```python
from build123d import *

# Parameters (mm, degrees)
SKETCH1_W           = 127
SKETCH1_H           = 127
BOSS_EXTRUDE1_DEPTH = 6.35
SKETCH2_W           = 50.8
SKETCH2_H           = 63.5
CUT_EXTRUDE1_DEPTH  = 180.717340566
SKETCH3_R           = 14.3002
CUT_EXTRUDE2_DEPTH  = 180.717340566
SKETCH5_R           = 2.5527
CUT_EXTRUDE4_DEPTH  = 180.717340566
CIRPATTERN1_COUNT   = 8
SKETCH6_R           = 14.3002
CUT_EXTRUDE5_DEPTH  = 180.717340566
FILLET1_R           = 2.54
FILLET2_R           = 25.4
SKETCH10_R          = 2.5527
CUT_EXTRUDE7_DEPTH  = 180.717340566
LPATTERN1_COUNT     = 5
LPATTERN1_PITCH     = 25.4


with BuildPart() as part:
    # Sketch1 → Boss-Extrude1 (new body)
    with BuildSketch(Plane(origin=(0, 0, 0), x_dir=(1, 0, 0), z_dir=(0, 1, 0))):
        with Locations((-63.5, 63.5)):
            Rectangle(SKETCH1_W, SKETCH1_H)
    extrude(amount=BOSS_EXTRUDE1_DEPTH)

    # Sketch2 → Cut-Extrude1 (cut, through all)
    with BuildSketch(Plane(origin=(0, 6.35, 0), x_dir=(1, 0, 0), z_dir=(0, 1, 0))):
        with Locations((-25.4, 95.25)):
            Rectangle(SKETCH2_W, SKETCH2_H)
    extrude(amount=-CUT_EXTRUDE1_DEPTH, mode=Mode.SUBTRACT)

    # Sketch3 → Cut-Extrude2 (cut, through all)
    with BuildSketch(Plane(origin=(0, 6.35, 0), x_dir=(1, 0, 0), z_dir=(0, 1, 0))):
        with Locations(Location((-38.1, 31.75, 0), (0, 0, 270))):
            Circle(SKETCH3_R)
    extrude(amount=-CUT_EXTRUDE2_DEPTH, mode=Mode.SUBTRACT)

    # Sketch5 → Cut-Extrude4 (cut, through all)
    with BuildSketch(Plane(origin=(0, 6.35, 0), x_dir=(1, 0, 0), z_dir=(0, 1, 0))):
        with Locations(Location((-114.3, 95.25, 0), (0, 0, 270))):
            Circle(SKETCH5_R)
    cut_extrude4 = extrude(amount=-CUT_EXTRUDE4_DEPTH, mode=Mode.SUBTRACT)

    # CirPattern1: Cut-Extrude4 ×8 about axis, 4 skipped
    cirpattern1_axis = Axis((-88.9, 6.35, -95.25), (0, 1, 0))
    add([cut_extrude4.rotate(cirpattern1_axis, i * 360 / CIRPATTERN1_COUNT) for i in range(1, CIRPATTERN1_COUNT) if i not in (1, 2, 5, 6)], mode=Mode.SUBTRACT)

    # Sketch6 → Cut-Extrude5 (cut, through all)
    with BuildSketch(Plane(origin=(0, 6.35, 0), x_dir=(1, 0, 0), z_dir=(0, 1, 0))):
        with Locations(Location((-88.9, 95.25, 0), (0, 0, 270))):
            Circle(SKETCH6_R)
    extrude(amount=-CUT_EXTRUDE5_DEPTH, mode=Mode.SUBTRACT)

    # Fillet1
    fillet1_edges = [part.edges().sort_by_distance(p)[0] for p in [
        (0, 3.175, -63.5),
        (-50.8, 3.175, -127),
        (0, 3.175, 0),
        (-127, 3.175, 0),
        (-127, 3.175, -127),
    ]]
    fillet(fillet1_edges, radius=FILLET1_R)

    # Fillet2
    fillet2_edges = [part.edges().sort_by_distance(p)[0] for p in [
        (-50.8, 3.175, -63.5),
    ]]
    fillet(fillet2_edges, radius=FILLET2_R)

    # Sketch10 → Cut-Extrude7 (cut, through all)
    with BuildSketch(Plane(origin=(0, 6.35, 0), x_dir=(1, 0, 0), z_dir=(0, 1, 0))):
        with Locations(Location((-107.95, 12.7, 0), (0, 0, 270))):
            Circle(SKETCH10_R)
    cut_extrude7 = extrude(amount=-CUT_EXTRUDE7_DEPTH, mode=Mode.SUBTRACT)

    # LPattern1: Cut-Extrude7 ×5, 1 skipped
    with Locations(*[(0, 0, -i * LPATTERN1_PITCH) for i in range(1, LPATTERN1_COUNT) if i not in (4,)]):
        add(cut_extrude7, mode=Mode.SUBTRACT)


solid = part.part
```
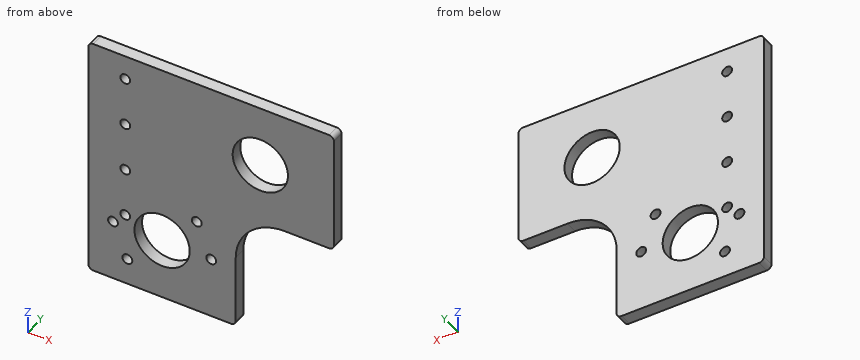
Source: CAD feature listing. Evaluate the final solid. Frame: model axes, mm. Give positions to 0.01 mm unless a question says otherwise; leave off trailing zeros. Loops run counter-clockwise (first coordinate to the right, second up) from the corner with the lowest first, then second, coordinate; pieces in that order, holes last. Notation, with made-up numbers: (84.5, -17.75) -> (126.5, -17.75) arc R29 cw to (126.5, 11.25) -> close; hole circle Ø5 at (68.5, 40.5). An arc over 180 degrees is marked (long way). Put each result on its own line as item: value. Start each with the question number.
1) Contact query for flat-ended pins moving along their axis: P1, Ø3, axis at x = -107.95, z = -88.9, coming from the -Y side; P2, Ø1.5, axis at y = 4.5, z = -106, coming from the +X side. Output: stop coordinate, or through.
2) Cut plane B-B (z = -31.75). Return loops of the section in (x, y), then the cut area to 3 significant figures.
3) Cut plane A-A (x = -88.9). Return loops of the section in (y, z).
4) Cut plane C-C (y = 3.5). State how many separate pieces and enclosed holes the cut face has, then the cut area to 3 significant figures.
5) Cut plane D-D (x = -19). Return loops of the section in (y, z).
6) Material intervals for probe 1 along X at (y, z) = (2, -95.25); probe 2 along Z at (x, y) = (-89.5, 5); probe 3 along Z at (x, y) = (-63.5, 2.5), sorted ascending.
Results are:
1. P1: passes through
1. P2: stops at x = -50.8
2. outline: (-127, 0) -> (-52.4, 0) -> (-52.4, 6.35) -> (-127, 6.35) -> close; (-23.8, 0) -> (0, 0) -> (0, 6.35) -> (-23.8, 6.35) -> close
2. area: 625 mm2
3. outline: (0, -127) -> (6.35, -127) -> (6.35, -109.55) -> (0, -109.55) -> close; (0, -80.95) -> (6.35, -80.95) -> (6.35, 0) -> (0, 0) -> close
4. separate pieces: 1
4. enclosed holes: 10
4. area: 11,600 mm2
5. outline: (0, -63.5) -> (6.35, -63.5) -> (6.35, 0) -> (0, 0) -> close
6. probe 1: x = -127 to -116.85, -111.75 to -103.2, -74.6 to -66.05, -60.95 to -50.8
6. probe 2: z = -127 to -109.54, -80.96 to 0
6. probe 3: z = -127 to -97.8, -92.7 to 0
